Build history of the part. All positions in model axes, mm. Face numbers are marked on the shaded views. A direction names the side the tool comes from. Round coordinates to 2 decimals unless told otherwise and drop trailing zeros. Order: outer loops, then holes, each group sorted by start corner. A loop starts at its lowest first (then second) coordinate and runs counter-clockwise, first axis right, second up. Notation, with made-up numbers: M 17,52 L 69,52 A8 ccw 69,56 Z; hole C -23.75,-38 d8. An arc over 180 degrees is marked long. One line per item, written item: value. Start each with the question number.
Item 1: Pin check, flat tips, straight feed: pin 1 (0.8 mm diameter, centred on x = 7.5, y = 6, fed in from -Z); pin 2 (1.8 mm diameter, centred on x = -10.5, z = -18, fed in from +Y); pin 3 (13.5 mm diameter, centred on x = 2.5, z = 3.5, fed in from +Y). Stop position of each tip, or through.
Item 2: Band-saw the part on B-B, the plane x = -8. Write the cut outline in (y, z), then the cut area to 3 significant figures.
Item 3: Band-saw the part on A-A, the plane z = 20.77. Write the cut outline in (x, y), then the cut area to 3 significant figures.
Item 4: Band-saw the part on D-D, the plane z = 13. Write the cut outline in (x, y).
Item 5: Two-plate mould, pull along X, no slides. Class the marked faces 5, 6, 7 and 8: +X half, -X half, draft (parallel to the pull), parting line (faces both ways), or undercut.
Item 6: Probe L1, parallel to X at y = 2.75, z = 29; L2, parallel to Z at x = 8, y = 1.8; L3, parallel to Z at x = 0, y = 3.5. List the from-to ranges inside material, lowest first.
Item 7: Tool access for the marked faces 1, 2, 3 and 4: list every direction of +Z, -Z, +X, -X, +Y, -Y with a clear straight run to the whole face (end or side of a thin tool).
Item 8: Band-saw the part on C-C, the plane x = -1. Write the cut outline in (y, z).
Autodesk Inventor part; units mm, degrees
ref_plane "YZ Plane" through (0, 0, 0) normal (1, 0, 0) x (0, 1, 0)
ref_plane "XZ Plane" through (0, 0, 0) normal (0, 1, 0) x (-1, 0, 0)
ref_plane "XY Plane" through (0, 0, 0) normal (0, 0, 1) x (1, 0, 0)
sketch "Sketch1" plane through (0, 0, 0) normal (0, 1, 0) x (-1, 0, 0)
  line L0 (15, 30.94) -> (-15, 30.94)
  line L1 (-15, 30.94) -> (-15, -21.4)
  line L2 (-15, -21.4) -> (15, -21.4)
  line L3 (15, -21.4) -> (15, 30.94)
  line L4 (0, 30.94) -> (0, -21.4) construction
  line L5 (15, 0) -> (-15, 0) construction
  line L6 (15, 4.77) -> (-15, 4.77) construction
  point P0 (0, 0)
  point P1 (0, 0)
  dimension "d0" = 52.34
  dimension "d1" = 30
  dimension "d64" = 4.77
extrude "Extrusion1" add sketch "Sketch1" along normal blind 6.25
sketch "Sketch2" plane through (0, 6.25, 0) normal (0, 1, 0) x (1, 0, 0)
  circle A0 centre (0, 0) radius 11 construction
  line L0 (0, 0) -> (-4.2095, -10.1627) construction
  line L1 (-15, -30.94) -> (15, -30.94)
  line L2 (15, -30.94) -> (15, 21.4)
  line L3 (15, 21.4) -> (-15, 21.4)
  line L4 (-15, 21.4) -> (-15, -30.94)
  line L5 (0, 0) -> (-4.2095, -10.1627) construction
  line L6 (0, 0) -> (0, -30.94) construction
  point P0 (4.2095, -10.1627)
  point P1 (10.1627, -4.2095)
  point P2 (10.1627, 4.2095)
  point P3 (4.2095, 10.1627)
  point P4 (-4.2095, 10.1627)
  point P5 (-10.1627, 4.2095)
  point P6 (-10.1627, -4.2095)
  dimension "d7" = 22
  dimension "d8" = 360
  dimension "d98" = 22.5
hole "Hole1" at (-4.2095, 6.25, 10.1627) at (-10.1627, 6.25, 4.2095) at (-10.1627, 6.25, -4.2095) at (-4.2095, 6.25, -10.1627) at (4.2095, 6.25, -10.1627) at (10.1627, 6.25, -4.2095) at (10.1627, 6.25, 4.2095) at (4.2095, 6.25, 10.1627) direction (0, -1, 0) diameter 2.5 end through all
sketch "Sketch3" plane through (0, 6.25, 0) normal (0, 1, 0) x (1, 0, 0)
  circle A0 centre (0, 0) radius 5.05
  dimension "d17" = 10.1
extrude "Extrusion2" cut sketch "Sketch3" against normal through all
sketch "Sketch4" plane through (0, 6.25, 0) normal (0, 1, 0) x (1, 0, 0)
  line L0 (-8, -20.77) -> (8, -20.77) construction
  line L1 (8, -20.77) -> (8, 11.23) construction
  line L2 (8, 11.23) -> (-8, 11.23) construction
  line L3 (-8, 11.23) -> (-8, -20.77) construction
  line L4 (-15, -30.94) -> (15, -30.94) construction
  line L5 (0, -30.94) -> (0, 21.4) construction
  line L6 (15, 21.4) -> (-15, 21.4) construction
  line L7 (-15, 21.4) -> (-15, -30.94) construction
  line L8 (-15, -4.77) -> (15, -4.77) construction
  line L9 (15, -30.94) -> (15, 21.4) construction
  line L10 (0, -20.77) -> (0, 11.23) construction
  line L11 (-8, -4.77) -> (8, -4.77) construction
  point P0 (0, 0)
  dimension "d20" = 32
  dimension "d21" = 16
hole "Hole2" at (-8, 6.25, 20.77) at (8, 6.25, 20.77) at (8, 6.25, -11.23) at (-8, 6.25, -11.23) direction (0, -1, 0) diameter 3 end through all
sketch "Sketch6" plane through (-15, 0, 30.94) normal (0, 0, 1) x (1, 0, 0)
  line L0 (-10.3797, 2.75) -> (37.9037, 2.75) construction
  line L1 (0, 0) -> (30, 0) construction
  line L2 (0, 0) -> (0, 6.25)
  point P0 (15, 0)
  point P1 (4.5, 2.75)
  point P2 (11.5, 2.75)
  point P3 (18.5, 2.75)
  point P4 (25.5, 2.75)
  dimension "d33" = 2.75
  dimension "d34" = 4.5
  dimension "d37" = 7
hole "Hole3" at (-10.5, 2.75, 30.94) at (-3.5, 2.75, 30.94) at (3.5, 2.75, 30.94) at (10.5, 2.75, 30.94) direction (0, 0, -1) diameter 2.013 depth 7.6 tip angle 118
sketch "Sketch7" plane through (15, 0, -21.4) normal (0, 0, -1) x (-1, 0, 0)
  line L0 (-10.51, 2.75) -> (37.7733, 2.75) construction
  line L1 (0, 0) -> (29.8697, 0) construction
  line L2 (0, 0) -> (0, 3.7534)
  line L3 (0, 0) -> (30, 0)
  line L4 (0, 0) -> (0, 6.25)
  point P0 (15, 0)
  point P1 (15, 0)
  point P2 (4.5, 2.75)
  point P3 (11.5, 2.75)
  point P4 (18.5, 2.75)
  point P5 (25.5, 2.75)
  dimension "d53" = 2.75
  dimension "d54" = 4.5
  dimension "d55" = 7
hole "Hole4" at (10.5, 2.75, -21.4) at (-10.5, 2.75, -21.4) at (-3.5, 2.75, -21.4) at (3.5, 2.75, -21.4) direction (0, 0, 1) diameter 2.013 depth 7.6 tip angle 118
sketch "Sketch8" plane through (0, 6.25, 0) normal (0, 1, 0) x (1, 0, 0)
  line L0 (0, 32.012) -> (0, -41.432) construction
  line L1 (-15, -30.94) -> (15, -30.94)
  line L2 (15, 21.4) -> (-15, 21.4)
  line L3 (-1.5, -30.94) -> (-15, -30.94)
  line L4 (-15, -30.94) -> (-15, -24.94)
  line L5 (-15, -24.94) -> (-1.5, -24.94)
  line L6 (1.5, -30.94) -> (15, -30.94)
  line L7 (15, -30.94) -> (15, -24.94)
  line L8 (15, -24.94) -> (1.5, -24.94)
  line L9 (15, -30.94) -> (15, 21.4)
  line L10 (-15, 21.4) -> (-15, -30.94)
  line L11 (-1.5, -24.94) -> (-1.5, -30.94)
  line L12 (-15, -30.94) -> (15, -30.94)
  line L13 (1.5, -24.94) -> (1.5, -30.94)
  line L14 (-15, -4.77) -> (15, -4.77) construction
  line L15 (-1.5, 21.4) -> (-15, 21.4)
  line L16 (-15, 21.4) -> (-15, 15.4)
  line L17 (-15, 15.4) -> (-1.5, 15.4)
  line L18 (1.5, 21.4) -> (15, 21.4)
  line L19 (15, 21.4) -> (15, 15.4)
  line L20 (15, 15.4) -> (1.5, 15.4)
  line L21 (-1.5, 15.4) -> (-1.5, 21.4)
  line L22 (1.5, 15.4) -> (1.5, 21.4)
  line L23 (-21.8515, -28.94) -> (23.2072, -28.94) construction
  point P0 (0, 0)
  dimension "d80" = 6
  dimension "d81" = 3
  dimension "d82" = 13.5
  dimension "d86" = 2
sketch "Sketch9" plane through (0, 6.25, 0) normal (0, 1, 0) x (1, 0, 0)
  circle A0 centre (-4.2095, -10.1627) radius 1.25 construction
  circle A1 centre (4.2095, -10.1627) radius 1.25 construction
  circle A2 centre (10.1627, -4.2095) radius 1.25 construction
  circle A3 centre (10.1627, 4.2095) radius 1.25 construction
  circle A4 centre (4.2095, 10.1627) radius 1.25 construction
  circle A5 centre (-4.2095, 10.1627) radius 1.25 construction
  circle A6 centre (-10.1627, 4.2095) radius 1.25 construction
  circle A7 centre (-10.1627, -4.2095) radius 1.25 construction
  circle A8 centre (0, 0) radius 11 construction
hole "Hole5" at (-4.2095, 6.25, 10.1627) at (4.2095, 6.25, 10.1627) at (10.1627, 6.25, 4.2095) at (10.1627, 6.25, -4.2095) at (4.2095, 6.25, -10.1627) at (-4.2095, 6.25, -10.1627) at (-10.1627, 6.25, -4.2095) at (-10.1627, 6.25, 4.2095) direction (0, -1, 0) diameter 5 depth 2.175
extrude "Extrusion6" cut sketch "Sketch8" against normal blind 0.75 contours L4 L5 L11 L1 | L13 L8 L7 L1 | L10 L2 L21 L17 | L20 L22 L2 L9
fillet "Fillet1" radius 3 4 edges at (1.5, 5.875, 24.94) (-1.5, 5.875, 24.94) (1.5, 5.875, -15.4) (-1.5, 5.875, -15.4)
sketch "Sketch11" plane through (0, 6.25, 0) normal (0, 1, 0) x (1, 0, 0)
  line L0 (-13.5, -23.44) -> (13.5, -23.44)
  line L1 (13.5, -23.44) -> (13.5, 13.9)
  line L2 (13.5, 13.9) -> (-13.5, 13.9)
  line L3 (-13.5, 13.9) -> (-13.5, -23.44)
  line L4 (-15, 15.4) -> (-15, -24.94)
  line L5 (15, -24.94) -> (15, 15.4)
  line L6 (-1.5, -30.94) -> (-15, -30.94)
  line L7 (-15, 21.4) -> (-1.5, 21.4)
  circle A0 centre (-8, 11.23) radius 3 construction
  arc A1 (-6.5016, 11.1609) -> (-6.6857, 10.5071) centre (-8, 11.23) ccw construction
  point P0 (0, 0)
  dimension "d87" = 7.5
  dimension "d88" = 7.5
  dimension "d91" = 1.5
  dimension "d92" = 1.5
  dimension "d93" = 6
extrude "Extrusion7" cut sketch "Sketch11" against normal blind 2.25
fillet "Fillet2" radius 1.5 4 edges at (-13.5, 5.125, 23.44) (13.5, 5.125, 23.44) (13.5, 5.125, -13.9) (-13.5, 5.125, -13.9)
equation "\"d0\" = total_width"
equation "\"d64\" = axis_offset"
equation "\"d3\" = plate_thickness"
equation "\"d7\" = d9"
equation "\"d18\" = plate_thickness"
equation "\"d33\" = hole_2_bottom"
equation "\"d53\" = hole_2_bottom"
equation "\"d83\" = plate_thickness - border_thickness"
equation "\"plate_thickness\" = 6.25"
equation "\"d9\" = 22"
equation "\"tol\" = 0.1"
equation "\"border_thickness\" = 5.5"
equation "\"hole_2_bottom\" = 0.5 * border_thickness"
equation "\"central_thickness\" = 4"
equation "\"side_thickness\" = 3"
equation "\"side_trace_depth\" = 1"
equation "\"internal_width\" = bloc_106_spacing - side_thickness"
equation "\"total_width\" = internal_width + 2 * side_trace_depth"
equation "\"axis_offset\" = 0.5 * internal_width + side_thickness - axis_to_N102"
equation "\"bloc_106_spacing\" = 53.34"
equation "\"axis_to_N102\" = 23.4"
properties part number "new_base_u64" material "Aluminum 2014-T4"
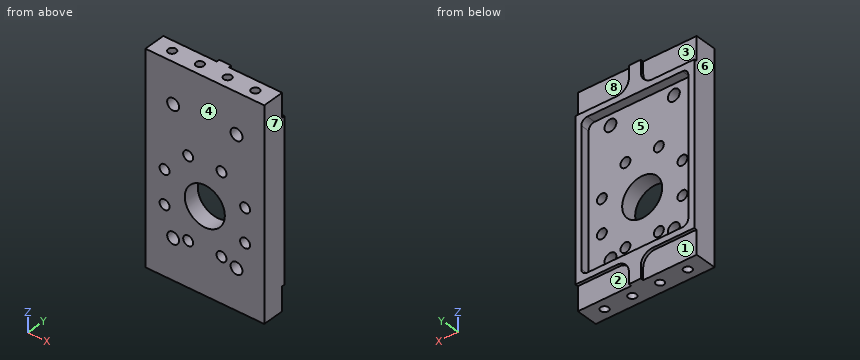
Output:
1. pin 1: stops at z = -15.4
1. pin 2: stops at y = 5.5
1. pin 3: stops at y = 4
2. outline: M 0,-21.4 L 5.5,-21.4 L 5.5,-15.4 L 6.25,-15.4 L 6.25,-13.9 L 4,-13.9 L 4,-12.73 L 0,-12.73 Z; M 0,-9.73 L 4,-9.73 L 4,19.27 L 0,19.27 Z; M 0,22.27 L 4,22.27 L 4,23.44 L 6.25,23.44 L 6.25,24.94 L 5.5,24.94 L 5.5,30.94 L 0,30.94 Z
2. area: 210 mm²
3. outline: M -15,0 L -9.5,0 L -9.5,4 L -13.5,4 L -13.5,6.25 L -15,6.25 Z; M -6.5,0 L 6.5,0 L 6.5,4 L -6.5,4 Z; M 9.5,0 L 15,0 L 15,6.25 L 13.5,6.25 L 13.5,4 L 9.5,4 Z
3. area: 103 mm²
4. outline: M -15,0 L 15,0 L 15,6.25 L 13.5,6.25 L 13.5,4 L -13.5,4 L -13.5,6.25 L -15,6.25 Z
5. face 5: undercut
5. face 6: -X half
5. face 7: +X half
5. face 8: draft
6. L1: x = -15 to -11.51, -9.49 to -4.51, -2.49 to 2.49, 4.51 to 9.49, 11.51 to 15
6. L2: z = -21.4 to -12.73, -9.73 to 19.27, 22.27 to 30.94
6. L3: z = -21.4 to -5.05, 5.05 to 30.94
7. face 1: -Z, -X, +Y
7. face 2: -Z, +X, +Y
7. face 3: +Z, -X, +Y
7. face 4: +Z, -Z, +X, -X, -Y
8. outline: M 0,-21.4 L 6.25,-21.4 L 6.25,-13.9 L 4,-13.9 L 4,-4.95 L 0,-4.95 Z; M 0,4.95 L 4,4.95 L 4,23.44 L 6.25,23.44 L 6.25,30.94 L 0,30.94 Z
